Answer from the drawing. Dimensions are ordinates in mm from the lowest x, y and z of the part. A direction names the side the tool comes from. Give positions to 0.01 mm unless a question says otherwise; leave off trailing zeros. Loops run counter-clockwise (first coordinate to the right, second up) from the corner with the lowest first, then second, coordinate; pieces in that order, holes last.
Item 1: A tool of negligible diameter and unlimited length cuts with its end or side. For the marked faces 1, 2 and 3, from which of +Z, -Z, +X, -X, +Y, -Y can it reach the whole face along a straight path? Write none if from no direction.
Item 2: Consider line 1 along Z through (x, y) = (99, 26.5); line 2 along X through (y, z) = (3, 10.5); line 3 along X through (y, z) = (34, 32.5). Determine where each line is inside the solid, lowest interval first.
Item 3: Section B-B, the plane y = 34 is taken. Give the vertices of the cut face in (x, z), and give its area (3 significant figures).
Item 4: The mould has two halves that part along Z. Classify the marked faces 4, 5, 6 and 7: pulls with the +Z half, pulls with the -Z half, needs draft (parallel to the pull), parting line crosses it, or undercut.
Item 5: Each of these flat-tipped pins is pushed along its axis until it touches: pin 1 Ø3 at (x, z) = (55.68, 23.94) entering from +Y; pin 2 Ø4 at (x, z) = (70.5, 36.5) entering from -Y (1 decimal); pin 3 Ø8 at (y, z) = (31.5, 36.5) entering from -X; pin 4 Ø8.5 at (x, z) = (17, 16.5) entering from +Y. Where does it stop, or does it pass through?
Item 6: Section D-D, the plane x = 26 is taken. Give the vertices of the cut face in (y, z), and give its area (3 significant figures).
Item 7: Section C-C, the plane z = 3 is taken. Give the vertices of the cut face in (x, y), and give its area (3 significant figures).
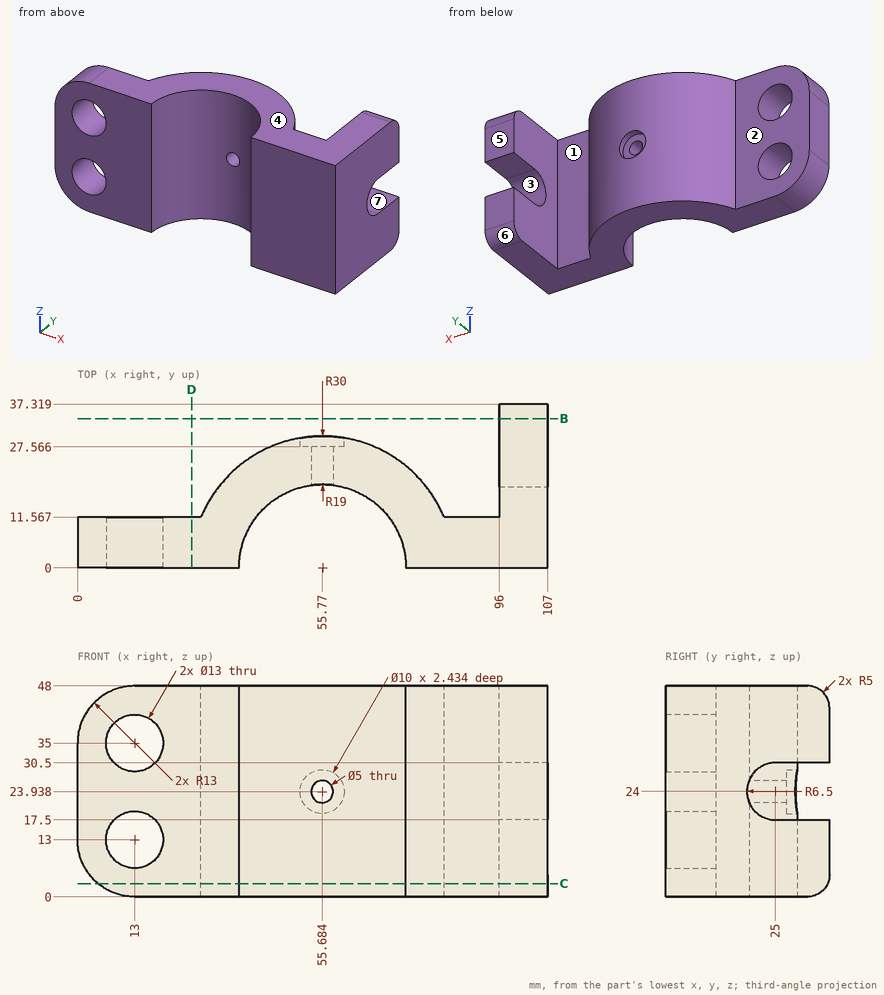
Worked answers:
1. face 1: +Z, -Z, +Y
1. face 2: +Z, -Z, -X, +Y
1. face 3: +X, +Y
2. line 1: z = 0 to 17.5, 30.5 to 48
2. line 2: x = 0.24 to 7, 19 to 37.01, 74.53 to 107
2. line 3: x = 96 to 107
3. outline: (96, 0.29) - (107, 0.29) - (107, 17.5) - (96, 17.5) - close; (96, 30.5) - (107, 30.5) - (107, 47.71) - (96, 47.71) - close
3. area: 379 mm2
4. face 4: pulls with the +Z half
4. face 5: needs draft
4. face 6: pulls with the -Z half
4. face 7: undercut
5. pin 1: passes through
5. pin 2: stops at y = 9
5. pin 3: stops at x = 43.78
5. pin 4: stops at y = 11.57
6. outline: (0, 0) - (11.57, 0) - (11.57, 48) - (0, 48) - close
6. area: 555 mm2
7. outline: (4.69, 0) - (36.77, 0) arc R19 cw to (74.77, 0) - (107, 0) - (107, 36.9) - (96, 36.9) - (96, 11.57) - (83.45, 11.57) arc R30 ccw to (28.09, 11.57) - (4.69, 11.57) - close
7. area: 1,630 mm2
